Geometry: final body of the model. Coordinates: model frame, mm. Face numbers are marked on the shaded views. Round coordinates to 2 decimals unless told otherwise and drop trailing zeros. Order: outer loops, then holes, each group sorted by start corner. A loop starts at its lowest first (then second) coordinate and runs counter-clockwise, first axis right, second up. Notation, with made-up numbers: M 53,62.25 L 59,62.25 A20 ccw 59,92.25 Z; hole C 34.25,-22 d11. An arc over 180 degrees is marked long. Put each result on its own line as item: value. Start each with the question number.
1) First-contact query: P1, Ø3, axis at x = -3, z = -2.5, coming from the -Y side. Flat tip, straight axial feed; report the tip coordinate or a pass-through.
2) Section B-B, the plane y = 0.6. Return loops of the section in (x, z).
3) Material intervals for probe 1 along X at (y, z) = (0.95, -3.5); probe 2 along Z at (x, y) = (8.5, 0.9); probe 3 along X at (y, z) = (0.45, -1.75), sorted ascending. Write a range as [from, to].
4) Section A-A, the plane z = -2.5. Return loops of the section in (x, y).
5) Draft query along X for the marked faces 1, 2, 3 and 4. Return one class per face: pulls with the +X half, pulls with the -X half, needs draft (parallel to the pull), parting line crosses it, or undercut.
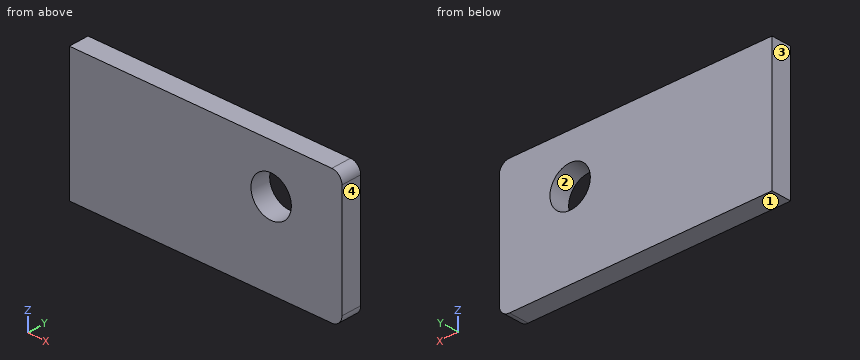
from build123d import *

# Parameters (mm, degrees)
SKETCH1_R           = 2
BOSS_EXTRUDE1_DEPTH = 2


with BuildPart() as part:
    # Sketch1 → Boss-Extrude1 (new body)
    with BuildSketch(Plane(origin=(0, 0, 0), x_dir=(1, 0, 0), z_dir=(0, 1, 0))):
        with BuildLine():
            Line((14.027461704, 3.38740458), (14.027461704, 10.632365856))
            ThreePointArc((14.027461704, 10.632365856), (13.733553665, 11.34192263), (13.023996891, 11.635830669))
            Line((13.023996891, 11.635830669), (-12.972538296, 11.635830669))
            Line((-12.972538296, 11.635830669), (-12.972538296, -1.364169331))
            Line((-12.972538296, -1.364169331), (13.023996891, -1.364169331))
            ThreePointArc((13.023996891, -1.364169331), (13.733553665, -1.070261292), (14.027461704, -0.360704518))
            Line((14.027461704, -0.360704518), (14.027461704, 3.38740458))
        make_face()
        with Locations(Location((7.015267176, 3.38740458, 0), (0, 0, 270))):
            Circle(SKETCH1_R, mode=Mode.SUBTRACT)
    extrude(amount=BOSS_EXTRUDE1_DEPTH)


solid = part.part
Result sheet:
1. P1: stops at y = 0
2. outline: M -12.97,-11.64 L 13.02,-11.64 A1 ccw 14.03,-10.63 L 14.03,0.36 A1 ccw 13.02,1.36 L -12.97,1.36 Z; hole C 7.02,-3.39 d4
3. probe 1: x = [-12.97, 5.02], [9.01, 14.03]
3. probe 2: z = [-11.64, -4.73], [-2.05, 1.36]
3. probe 3: x = [-12.97, 5.87], [8.16, 14.03]
4. outline: M -12.97,0 L 5.22,0 L 5.22,2 L -12.97,2 Z; M 8.81,0 L 14.03,0 L 14.03,2 L 8.81,2 Z
5. face 1: needs draft
5. face 2: undercut
5. face 3: pulls with the -X half
5. face 4: pulls with the +X half
